Work out the finished part from the listing and answer in its coordinate system (mm). A direction names the side the tool comes from. Give positions to 0.01 mm unless a question says otherwise; leave off trailing zeros. Loops run counter-clockwise (first coordinate to the right, second up) from the corner with the lowest first, then second, coordinate; pieces in that order, holes last. Notation, with made-up numbers: (-26.75, 22.25) - (16.25, 22.25) arc R16 cw to (16.25, 49.25) - close; hole circle Ø5 at (89.25, -34.75). An arc over 180 degrees is marked (long way). One line per question, with ' | ' between items. Start each with the question number.
1. Find the intervals of material crossed by line 1 (Z direction, x = 3.75, y = 5); line 2 (Y direction, x = 0, z = 7.25); line 3 (X direction, y = 0, z = 6.75), in increasing order.
2. For a pull along Y with two mould halves and no side action, classify faces 1 (the face through (5.262, 6.862, 5.698)), 2 (the face through (0, 0, 0)), 3 (the face through (-5.44, -9.56, 4.93)) as released by +Y, released by -Y, zero draft, split by the parting line, or undercut.
3. Which of the six approach directions +Z, -Z, +X, -X, +Y, -Y give full straight-line access (tool end or side, diameter ignored) to faces 4 (the face through (5.56, -9.49, 4.93)), 5 (the face through (0, 0, 2))?
4. Section C-C (y = 10.75) is taken. Determine the outline of the cut face in (x, z).
5. Section D-D (y = -10.5) is taken. Determine the outline of the cut face in (x, z).
6. Section A-A (z = 2.5) is taken. Determine the outline of the cut face in (x, y).
7. Each of these flat-tipped pins is pushed along its axis until it touches: pin 1 (8.5 mm diameter, centred on x = 3, y = -0.5, fed in from +Z); pin 2 (3 mm diameter, centred on x = -2, z = 4.5, fed in from -Y); pin 3 (6 mm diameter, centred on x = 7.5, z = 2.5, fed in from -Y). Where does it stop, or does it pass through?
8. Section B-B (y = 0) is taken. Determine the outline of the cut face in (x, z).
Autodesk Inventor part; units mm, degrees
ref_plane "YZ Plane" through (0, 0, 0) normal (1, 0, 0) x (0, 1, 0)
ref_plane "XZ Plane" through (0, 0, 0) normal (0, 1, 0) x (-1, 0, 0)
ref_plane "XY Plane" through (0, 0, 0) normal (0, 0, 1) x (1, 0, 0)
sketch "Skizze1" plane through (0, 0, 0) normal (0, 0, 1) x (1, 0, 0)
  line L0 (-15.4146, 0) -> (15.4146, 0)
  line L1 (0, -17.7824) -> (0, 17.7824)
  line L2 (-10.9895, 6.3689) -> (0.0209, 12.7017)
  line L3 (0.0209, 12.7017) -> (11.0104, 6.3328)
  line L4 (11.0104, 6.3328) -> (10.9895, -6.3689)
  line L5 (10.9895, -6.3689) -> (-0.0209, -12.7017)
  line L6 (-0.0209, -12.7017) -> (-11.0104, -6.3328)
  line L7 (-11.0104, -6.3328) -> (-10.9895, 6.3689)
  circle A0 centre (0, 0) radius 10
  dimension "d0" = 20
  dimension "d1" = 11
extrude "Extrusion1" add sketch "Skizze1" along normal blind 10
sketch "Skizze2" plane through (0, 0, 10) normal (0, 0, 1) x (1, 0, 0)
  point P0 (0, 0)
hole "Bohrung1" at (0, 0, 10) direction (0, 0, -1) diameter 17.294 depth 8
chamfer "Fase1" distance 0.5 angle 45 1 edges at (0, 8.647, 10)
properties part number "Wasserverteiler2"
Conclusion:
1) line 1: 0 to 2 | line 2: -12.69 to -8.65, 8.65 to 12.69 | line 3: -11 to -8.65, 8.65 to 11
2) face 1: undercut | face 2: zero draft | face 3: released by -Y
3) face 4: +Z, -Z, +X, -Y | face 5: +Z
4) outline: (-3.37, 0) - (3.39, 0) - (3.39, 10) - (-3.37, 10) - close
5) outline: (-3.82, 0) - (3.81, 0) - (3.81, 10) - (-3.82, 10) - close
6) outline: (-11.01, -6.33) - (-0.02, -12.7) - (10.99, -6.37) - (11.01, 6.33) - (0.02, 12.7) - (-10.99, 6.37) - close; hole circle Ø17.29 at (0, 0)
7) pin 1: z = 2 | pin 2: y = -12.42 | pin 3: y = -10.1
8) outline: (-11, 0) - (11, 0) - (11, 10) - (9.15, 10) - (8.65, 9.5) - (8.65, 2) - (-8.65, 2) - (-8.65, 9.5) - (-9.15, 10) - (-11, 10) - close
